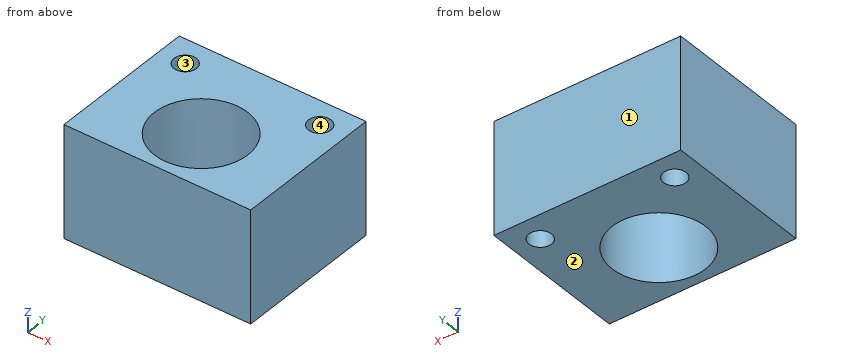
```python
from build123d import *

# Parameters (mm, degrees)
CROQUIS1_W              = 50
CROQUIS1_H              = 40
CROQUIS1_R              = 12.5
SALIENTE_EXTRUIR1_DEPTH = 30
CROQUIS2_R              = 3
CORTAR_EXTRUIR1_DEPTH   = 30
SALIENTE_EXTRUIR2_START = -30
CROQUIS3_R              = 12.5
SALIENTE_EXTRUIR2_DEPTH = 30
CROQUIS4_R              = 12.5
CORTAR_EXTRUIR2_DEPTH   = 20.1
CROQUIS5_R              = 12.5
CORTAR_EXTRUIR3_DEPTH   = 9.9


with BuildPart() as part:
    # Croquis1 → Saliente-Extruir1 (new body)
    with BuildSketch(Plane.XY):
        Rectangle(CROQUIS1_W, CROQUIS1_H)
        Circle(CROQUIS1_R, mode=Mode.SUBTRACT)
    extrude(amount=SALIENTE_EXTRUIR1_DEPTH)

    # Croquis2 → Cortar-Extruir1 (cut)
    with BuildSketch(Plane.XY.offset(30)):
        with Locations((-18, 13)):
            Circle(CROQUIS2_R)
        with Locations(Location((18, 13, 0), (0, 0, 180))):
            Circle(CROQUIS2_R)
    extrude(amount=-CORTAR_EXTRUIR1_DEPTH, mode=Mode.SUBTRACT)

    # Croquis3 → Saliente-Extruir2 (add)
    with BuildSketch(Plane.XY.offset(30).offset(SALIENTE_EXTRUIR2_START)):
        Circle(CROQUIS3_R)
    extrude(amount=SALIENTE_EXTRUIR2_DEPTH)

    # Croquis4 → Cortar-Extruir2 (cut)
    with BuildSketch(Plane.XY.offset(30)):
        with Locations((0, -4.809057324)):
            Circle(CROQUIS4_R)
    extrude(amount=-CORTAR_EXTRUIR2_DEPTH, mode=Mode.SUBTRACT)

    # Croquis5 → Cortar-Extruir3 (cut)
    with BuildSketch(Plane.XY.offset(9.9)):
        with Locations((0, -4.809057324)):
            Circle(CROQUIS5_R)
    extrude(amount=-CORTAR_EXTRUIR3_DEPTH, mode=Mode.SUBTRACT)


solid = part.part
```
Verification items for the finished model (mm, model axes). Face numbers are marked on the shaded views. Coordinates: 2 decimals unless noted, no trailing zeros. Order: outer loops, then holes, each group sorted by start corner. A loop starts at its lowest first (then second) coordinate and runs counter-clockwise, first axis right, second up. Notation, with made-up numbers: (-28.5, 47) -> (-16.5, 47) arc R30 cw to (-16.5, 76) -> close; hole circle Ø4 at (32, -7). An arc over 180 degrees is marked (long way). Put each result on its own line as item: value. Start each with the question number.
1) Cross-section at B-B (x = 0). Enter the section's corners in (y, z).
2) Cross-section at C-C (y = -3). Enter the section's corners in (x, z), plus the area to 3 significant figures.
3) Release check for a two-part mould opening along Y. For the marked faces 1, 2, 3 and 4 record: pulls with the +Y half, pulls with the -Y half, needs draft (parallel to the pull), parting line crosses it, or undercut.
4) Cross-section at A-A (y = 13). Enter the section's corners in (x, z), plus the area to 3 significant figures.
5) Material ranges on L1, parallel to Y at x = 0, z = 17; L2, parallel to Y at x = -18, z = 20; L3, parallel to X at y = 13.5, z = 8.25, recorded low to high.
6) Cross-section at D-D (z = 25.25). Enter the section's corners in (x, y), plus the area to 3 significant figures.
7) Go/stop test with a flat-tipped pin: pin 1 (15 mm diameter, centred on x = 0, y = -4.81, fed in from -Z). Record where the tip stops, or that it passes through.
Geometry check:
1. outline: (-20, 0) -> (-17.31, 0) -> (-17.31, 30) -> (-20, 30) -> close; (7.69, 0) -> (20, 0) -> (20, 30) -> (7.69, 30) -> close
2. outline: (-25, 0) -> (-12.37, 0) -> (-12.37, 30) -> (-25, 30) -> close; (12.37, 0) -> (25, 0) -> (25, 30) -> (12.37, 30) -> close
2. area: 758 mm^2
3. face 1: pulls with the +Y half
3. face 2: needs draft
3. face 3: undercut
3. face 4: undercut
4. outline: (-25, 0) -> (-21, 0) -> (-21, 30) -> (-25, 30) -> close; (-15, 0) -> (15, 0) -> (15, 30) -> (-15, 30) -> close; (21, 0) -> (25, 0) -> (25, 30) -> (21, 30) -> close
4. area: 1,140 mm^2
5. L1: y = -20 to -17.31, 7.69 to 20
5. L2: y = -20 to 10, 16 to 20
5. L3: x = -25 to -20.96, -15.04 to 15.04, 20.96 to 25
6. outline: (-25, -20) -> (25, -20) -> (25, 20) -> (-25, 20) -> close; hole circle Ø6 at (-18, 13); hole circle Ø25 at (0, -4.81); hole circle Ø6 at (18, 13)
6. area: 1,450 mm^2
7. pin 1: passes through
